Build history of the part. All positions in model axes, mm. Coordinates: 2 decimals unless noted, no trailing zeros. Loops run counter-clockwise (first coordinate to the right, second up) from the corner with the lowest first, then second, coordinate; pieces in that order, holes last. Notation, with made-up numbers: (63, 3.25) - (84, 3.25) arc R18 ccw to (84, 35.25) - close; hole circle Ø10 at (86, 50). An arc over 180 degrees is marked (long way). One line per item, written item: value.
```python
from build123d import *

# Parameters (mm, degrees)
SKETCH1_W            = 25.42
SKETCH1_H            = 25.42
BOSS_EXTRUDE5_DEPTH  = 4.7625
SKETCH3_W            = 4.7625
SKETCH3_H            = 61
BOSS_EXTRUDE6_DEPTH  = 1.27
SKETCH4_W            = 4.7625
SKETCH4_H            = 61
BOSS_EXTRUDE9_DEPTH  = 1.27
SKETCH6_W            = 63.54
SKETCH6_H            = 4.7625
BOSS_EXTRUDE10_DEPTH = 1.27
SKETCH7_W            = 63.54
SKETCH7_H            = 4.7625
BOSS_EXTRUDE11_DEPTH = 1.27


with BuildPart() as part:
    # Sketch1 → Boss-Extrude5 (new body)
    with BuildSketch(Plane.XY):
        with BuildLine():
            Line((0, 28.3), (0, 30.5))
            Line((0, 30.5), (-5.08, 30.5))
            Line((-5.08, 30.5), (-5.08, 5.08))
            Line((-5.08, 5.08), (0, 5.08))
            Line((0, 5.08), (0, 21.7))
            ThreePointArc((0, 21.7), (-3.3, 25), (0, 28.3))
        make_face()
        with BuildLine():
            Line((5.08, 30.5), (0, 30.5))
            Line((0, 30.5), (0, 28.3))
            ThreePointArc((0, 28.3), (2.333452378, 27.333452378), (3.3, 25))
            ThreePointArc((3.3, 25), (2.333452378, 22.666547622), (0, 21.7))
            Line((0, 21.7), (0, 5.08))
            Line((0, 5.08), (5.08, 5.08))
            Line((5.08, 5.08), (5.08, 30.5))
        make_face()
        with BuildLine():
            Line((30.5, 5.08), (5.08, 5.08))
            Line((5.08, 5.08), (5.08, 2.171785995))
            ThreePointArc((5.08, 2.171785995), (6.282811882, 1.369173548), (6.7479, 0))
            Line((6.7479, 0), (22.2521, 0))
            ThreePointArc((22.2521, 0), (24.5, 2.2479), (26.7479, 0))
            Line((26.7479, 0), (30.5, 0))
            Line((30.5, 0), (30.5, 5.08))
        make_face()
        with BuildLine():
            Line((22.2521, 0), (6.7479, 0))
            ThreePointArc((6.7479, 0), (6.282811882, -1.369173548), (5.08, -2.171785995))
            Line((5.08, -2.171785995), (5.08, -5.08))
            Line((5.08, -5.08), (30.5, -5.08))
            Line((30.5, -5.08), (30.5, 0))
            Line((30.5, 0), (26.7479, 0))
            ThreePointArc((26.7479, 0), (24.5, -2.2479), (22.2521, 0))
        make_face()
        with BuildLine():
            Line((2.2521, 0), (0, 0))
            Line((0, 0), (0, -5.08))
            Line((0, -5.08), (5.08, -5.08))
            Line((5.08, -5.08), (5.08, -2.171785995))
            ThreePointArc((5.08, -2.171785995), (3.130826452, -1.782811882), (2.2521, 0))
        make_face()
        with BuildLine():
            Line((0, -5.08), (0, 0))
            Line((0, 0), (-2.2521, 0))
            ThreePointArc((-2.2521, 0), (-3.130826452, -1.782811882), (-5.08, -2.171785995))
            Line((-5.08, -2.171785995), (-5.08, -5.08))
            Line((-5.08, -5.08), (0, -5.08))
        make_face()
        with BuildLine():
            Line((5.08, 2.171785995), (5.08, 5.08))
            Line((5.08, 5.08), (0, 5.08))
            Line((0, 5.08), (0, 0))
            Line((0, 0), (2.2521, 0))
            ThreePointArc((2.2521, 0), (3.130826452, 1.782811882), (5.08, 2.171785995))
        make_face()
        with BuildLine():
            Line((0, 5.08), (-5.08, 5.08))
            Line((-5.08, 5.08), (-5.08, 2.171785995))
            ThreePointArc((-5.08, 2.171785995), (-3.130826452, 1.782811882), (-2.2521, 0))
            Line((-2.2521, 0), (0, 0))
            Line((0, 0), (0, 5.08))
        make_face()
        with BuildLine():
            Line((-5.08, 2.171785995), (-5.08, 5.08))
            Line((-5.08, 5.08), (-30.5, 5.08))
            Line((-30.5, 5.08), (-30.5, 0))
            Line((-30.5, 0), (-26.7479, 0))
            ThreePointArc((-26.7479, 0), (-24.5, 2.2479), (-22.2521, 0))
            Line((-22.2521, 0), (-6.7479, 0))
            ThreePointArc((-6.7479, 0), (-6.282811882, 1.369173548), (-5.08, 2.171785995))
        make_face()
        with BuildLine():
            ThreePointArc((-5.08, -2.171785995), (-6.282811882, -1.369173548), (-6.7479, 0))
            Line((-6.7479, 0), (-22.2521, 0))
            ThreePointArc((-22.2521, 0), (-24.5, -2.2479), (-26.7479, 0))
            Line((-26.7479, 0), (-30.5, 0))
            Line((-30.5, 0), (-30.5, -5.08))
            Line((-30.5, -5.08), (-5.08, -5.08))
            Line((-5.08, -5.08), (-5.08, -2.171785995))
        make_face()
        with BuildLine():
            Line((0, -21.7), (0, -5.08))
            Line((0, -5.08), (-5.08, -5.08))
            Line((-5.08, -5.08), (-5.08, -30.5))
            Line((-5.08, -30.5), (0, -30.5))
            Line((0, -30.5), (0, -28.3))
            ThreePointArc((0, -28.3), (-3.3, -25), (0, -21.7))
        make_face()
        with BuildLine():
            Line((5.08, -5.08), (0, -5.08))
            Line((0, -5.08), (0, -21.7))
            ThreePointArc((0, -21.7), (2.333452378, -22.666547622), (3.3, -25))
            ThreePointArc((3.3, -25), (2.333452378, -27.333452378), (0, -28.3))
            Line((0, -28.3), (0, -30.5))
            Line((0, -30.5), (5.08, -30.5))
            Line((5.08, -30.5), (5.08, -5.08))
        make_face()
        with Locations((-17.79, 17.79)):
            Rectangle(SKETCH1_W, SKETCH1_H)
        with Locations((17.79, 17.79)):
            Rectangle(SKETCH1_W, SKETCH1_H)
        with Locations((17.79, -17.79)):
            Rectangle(SKETCH1_W, SKETCH1_H)
        with Locations((-17.79, -17.79)):
            Rectangle(SKETCH1_W, SKETCH1_H)
    extrude(amount=BOSS_EXTRUDE5_DEPTH)

    # Sketch3 → Boss-Extrude6 (add)
    with BuildSketch(Plane.ZY.offset(30.5)):
        with Locations((2.38125, 0)):
            Rectangle(SKETCH3_W, SKETCH3_H)
    extrude(amount=BOSS_EXTRUDE6_DEPTH)

    # Sketch4 → Boss-Extrude9 (add)
    with BuildSketch(Plane(origin=(30.5, 0, 0), x_dir=(0, 0, -1), z_dir=(1, 0, 0))):
        with Locations((-2.38125, 0)):
            Rectangle(SKETCH4_W, SKETCH4_H)
    extrude(amount=BOSS_EXTRUDE9_DEPTH)

    # Sketch6 → Boss-Extrude10 (add)
    with BuildSketch(Plane.XZ.offset(30.5)):
        with Locations((0, 2.38125)):
            Rectangle(SKETCH6_W, SKETCH6_H)
    extrude(amount=BOSS_EXTRUDE10_DEPTH)

    # Sketch7 → Boss-Extrude11 (add)
    with BuildSketch(Plane(origin=(0, 30.5, 0), x_dir=(1, 0, 0), z_dir=(0, 1, 0))):
        with Locations((0, -2.38125)):
            Rectangle(SKETCH7_W, SKETCH7_H)
    extrude(amount=BOSS_EXTRUDE11_DEPTH)


solid = part.part
```
Item 1: Cut at B-B, the plane z = 2.85. Write the cut outline in (x, y), then the cut area to 3 significant figures.
Check result:
outline: (-31.77, -31.77) - (31.77, -31.77) - (31.77, 31.77) - (-31.77, 31.77) - close; hole circle Ø4.5 at (-24.5, 0); hole circle Ø4.5 at (-4.5, 0); hole circle Ø6.6 at (0, -25); hole circle Ø6.6 at (0, 25); hole circle Ø4.5 at (4.5, 0); hole circle Ø4.5 at (24.5, 0)
area: 3,910 mm^2
Item 2: Cut at C-C, the plane x = -26. Write the cut outline in (y, z), then the cut area to 3 significant figures.
Check result:
outline: (-31.77, 0) - (-1.67, 0) - (-1.67, 4.76) - (-31.77, 4.76) - close; (1.67, 0) - (31.77, 0) - (31.77, 4.76) - (1.67, 4.76) - close
area: 287 mm^2
Item 3: Pull direction Y, two halves, no side cores. Call faces 1 (the face through (0, 0, 4.762)), 2 (the face through (0, 31.77, 2)), 3 (the face through (22.254, -0.099, 2.348)): released by +Y, released by -Y, zero draft, split by the parting line, or undercut.
Check result:
face 1: zero draft
face 2: released by +Y
face 3: undercut
Item 4: Cut at A-A, the plane x = 24.5. Write the cut outline in (y, z).
Check result:
outline: (-31.77, 0) - (-2.25, 0) - (-2.25, 4.76) - (-31.77, 4.76) - close; (2.25, 0) - (31.77, 0) - (31.77, 4.76) - (2.25, 4.76) - close
Item 5: Probe probe 1 along Y at (x, z) = (24.5, 1); probe 2 along X at (y, z) = (-25, 2.6); probe 3 along Y at (x, z) = (-23.5, 1.55). List the from-to ranges inside material, lowest first. Write a range as from..to.
Check result:
probe 1: y = -31.77..-2.25, 2.25..31.77
probe 2: x = -31.77..-3.3, 3.3..31.77
probe 3: y = -31.77..-2.01, 2.01..31.77
